from build123d import *

# Parameters (mm, degrees)
SKETCH1_R               = 43
SKETCH1_R_2             = 33.5
BOSS_EXTRUDE1_DEPTH     = 4.5
CUT_EXTRUDE1_START      = -5.5
CUT_EXTRUDE1_DEPTH      = 6.5
SKETCH3_R               = 2.025
CUT_EXTRUDE2_DEPTH      = 1
CUT_EXTRUDE2_DEPTH_BACK = 5.5


with BuildPart() as part:
    # Sketch1 → Boss-Extrude1 (new body)
    with BuildSketch(Plane(origin=(0, 0, 0), x_dir=(1, 0, 0), z_dir=(0, 1, 0))):
        Circle(SKETCH1_R)
        Circle(SKETCH1_R_2, mode=Mode.SUBTRACT)
    extrude(amount=BOSS_EXTRUDE1_DEPTH)

    # Sketch2 → Cut-Extrude1 (cut)
    with BuildSketch(Plane(origin=(0, 4.5, 0), x_dir=(1, 0, 0), z_dir=(0, 1, 0)).offset(CUT_EXTRUDE1_START)):
        with BuildLine():
            Line((0, 0), (0, -52.31984462))
            ThreePointArc((0, -52.31984462), (51.524988618, -9.085245674), (17.894440756, 49.16457191))
            Line((17.894440756, 49.16457191), (0, 0))
        make_face()
    cut_extrude1 = extrude(amount=CUT_EXTRUDE1_DEPTH, mode=Mode.SUBTRACT)

    # Mirror1: Cut-Extrude1 across plane
    add(cut_extrude1.mirror(Plane(origin=(0, 0, 0), x_dir=(0, 0, 1), z_dir=(1, 0, 0))), mode=Mode.SUBTRACT)

    # Sketch3 → Cut-Extrude2 (cut, two sides)
    with BuildSketch(Plane(origin=(0, 4.5, 0), x_dir=(1, 0, 0), z_dir=(0, 1, 0))) as cut_extrude2_sk:
        with Locations((0, 38)):
            Circle(SKETCH3_R)
    extrude(amount=CUT_EXTRUDE2_DEPTH, mode=Mode.SUBTRACT)
    extrude(cut_extrude2_sk.sketch, amount=-CUT_EXTRUDE2_DEPTH_BACK, mode=Mode.SUBTRACT)


solid = part.part
Source: CAD feature listing. Evaluate the final solid. Frame: model axes, mm. Give positions to 0.01 mm unless a question says otherwise; leave off trailing zeros. Write each loop counter-clockwise with the first axis right and the second up, starting at its lowest first coordinate (ties: lowest second). Pieces come first, ordered by that corner, then holes. Notation, with made-up numbers: M 18.25,26.25 L 24.25,26.25 A12 cw 24.25,43.25 Z; hole C -33.75,72.25 d2. An arc over 180 degrees is marked long. Return JSON: item names as keys, results as strings. Group by question number.
1) Ray query, L1, parallel to X at y = 2, z = -38 (3 decimals); L2, parallel to X at y = 1.95, z = -37; L3, parallel to Z at x = -1.25, y = 1.2. Return the intervals inside material, ascending.
2) First-contact query: pin 1 Ø1.5 at (y, z) = (1, -36.5) entering from +X. Flat tip, straight axial feed; report the tip coordinate or a pass-through.
3) Cut plane A-A, the plane x = 0. Output: boundary loops of the cut face in (y, z) (3 decimals).
4) Cut plane B-B, the plane y = 3.2. Output: boundary loops of the cut face in (x, z) (3 decimals), then the cut area to 3 significant figures.
5) Cut plane D-D, the plane x = -8.25. Output: boundary loops of the cut face in (y, z), then the cut area to 3 significant figures.
6) Draft query along X for faces 1 (the face through (1.1, 2.3, -39.7)), 2 (the face through (-13.105, 2.218, -36.006)), 3 (the face through (13.105, 2.218, -36.006)). Return one class per face: released by +X, released by -X, zero draft, split by the parting line, or undercut.
7) Cut plane C-C, the plane z = -32.5. Output: boundary loops of the cut face in (x, y).
Data:
{
 "1": {"L1": "x = -13.831 to -2.025, 2.025 to 13.831", "L2": "x = -13.47 to -1.76, 1.76 to 13.47", "L3": "z = -42.98 to -39.59, -36.41 to -33.48"},
 "2": {"pin 1": "stops at x = 13.56"},
 "3": {"outline": "M 0,-43 L 4.5,-43 L 4.5,-40.025 L 0,-40.025 Z; M 0,-35.975 L 4.5,-35.975 L 4.5,-33.5 L 0,-33.5 Z"},
 "4": {"outline": "M -14.707,-40.407 A43 ccw 14.707,-40.407 L 11.458,-31.48 A33.5 cw -11.458,-31.48 Z; hole C 0,-38 d4.05", "area": "241 mm²"},
 "5": {"outline": "M 0,-42.2 L 4.5,-42.2 L 4.5,-32.47 L 0,-32.47 Z", "area": "43.8 mm²"},
 "6": {"face 1": "undercut", "face 2": "released by -X", "face 3": "released by +X"},
 "7": {"outline": "M -11.83,0 L -8.12,0 L -8.12,4.5 L -11.83,4.5 Z; M 8.12,0 L 11.83,0 L 11.83,4.5 L 8.12,4.5 Z"}
}
